```python
from build123d import *

# Parameters (mm, degrees)
F0_R     = 16
F0_R_2   = 6
F1_DEPTH = 5.5
F2_R     = 12
F3_DEPTH = 2
F4_SIZE  = 3
F5_SIZE  = 0.5


with BuildPart() as f1:
    # F0 (on Top) → F1 (new body)
    with BuildSketch(Plane.XY):
        Circle(F0_R)
        Circle(F0_R_2, mode=Mode.SUBTRACT)
    extrude(amount=F1_DEPTH)

    # F2 (on face) → F3 (cut)
    with BuildSketch(Plane.XY.offset(5.5)):
        Circle(F2_R)
    extrude(amount=-F3_DEPTH, mode=Mode.SUBTRACT)

    # F4
    f4_edges = [f1.edges().sort_by_distance(p)[0] for p in [
        (-16, 0, 5.5),
    ]]
    chamfer(f4_edges, length=F4_SIZE)

    # F5
    f5_edges = [f1.edges().sort_by_distance(p)[0] for p in [
        (-16, 0, 0),
        (-6, 0, 0),
        (-6, 0, 3.5),
    ]]
    chamfer(f5_edges, length=F5_SIZE)


solid = f1.part
```
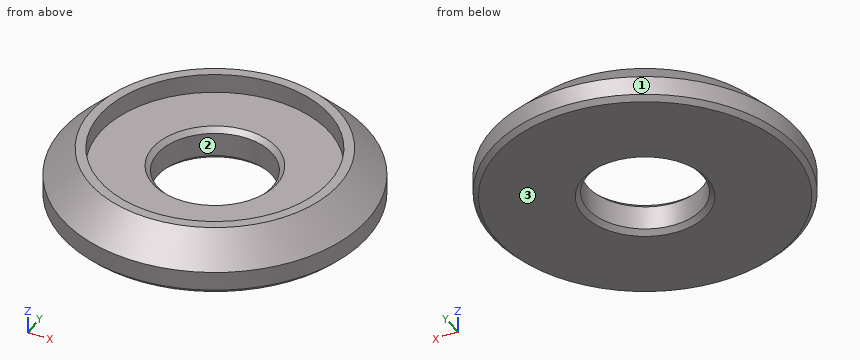
For this review, take the finished solid that the model builds, in its own axes (mm). Face numbers are marked on the shaded views. Coordinates: 2 decimals unless noted, no trailing zeros. Order: outer loops, then holes, each group sorted by start corner. A loop starts at its lowest first (then second) coordinate and runs counter-clockwise, first axis right, second up. Notation, with made-up numbers: (-30, 58) - (-12, 58) arc R21 ccw to (-12, 81) - close; hole circle Ø5 at (46.5, 1.5). An arc over 180 degrees is marked (long way). Answer as a JSON object with one key per item and string values. Group by question number.
1. We need section A-A on y = 0. State the section outline as (x, z) points, then the cut area to 4 significant figures.
2. We need section C-C on z = 5.1. State the section outline as (x, y) points.
3. Clearance check with a flat-ended pin moving along its axis: P1, Ø14.5, axis at x = 0, y = 0, coming from the +Z side. State where the tip first meets the part, or that it passes through.
4. The part is to be moulded in two halves that separate along Y. For the marked faces 1, 2 and 3, say which applies: pulls with the +Y half, pulls with the -Y half, needs draft (parallel to the pull), parting line crosses it, or undercut.
5. For probe 1 along Y at (x, z) = (0, 1.4); probe 2 along Z at (x, y) = (7, -1.5); probe 3 along Y at (x, z) = (-1, 2.3), list the stretches that pass through material, from the lowest coordinate up.
Final values:
{
 "1": {"outline": "(-16, 0.5) - (-15.5, 0) - (-6.5, 0) - (-6, 0.5) - (-6, 3) - (-6.5, 3.5) - (-12, 3.5) - (-12, 5.5) - (-13, 5.5) - (-16, 2.5) - close; (6, 0.5) - (6.5, 0) - (15.5, 0) - (16, 0.5) - (16, 2.5) - (13, 5.5) - (12, 5.5) - (12, 3.5) - (6.5, 3.5) - (6, 3) - close", "area": "76.25 mm²"},
 "2": {"outline": "circle Ø26.8 at (0, 0); hole circle Ø24 at (0, 0)"},
 "3": {"P1": "z = 3.5"},
 "4": {"face 1": "parting line crosses it", "face 2": "undercut", "face 3": "needs draft"},
 "5": {"probe 1": "-16 to -6, 6 to 16", "probe 2": "0 to 3.5", "probe 3": "-15.97 to -5.92, 5.92 to 15.97"}
}
